from build123d import *

# Parameters (mm, degrees)
EXTRU_MINCE1_DEPTH      = 280
ESQUISSE2_R             = 1.5
ENL_V_MAT_EXTRU_1_DEPTH = 281.847489752
ESQUISSE3_R             = 1.5
ENL_V_MAT_EXTRU_2_DEPTH = 282.354758268
CONG_1_R                = 5


with BuildPart() as part:
    # Esquisse1 → Extru.-Mince1 (new body)
    with BuildSketch(Plane.XY):
        Polygon((-9.75, 19.5), (-9.75, 0), (9.75, 0), (9.75, 19.5), (8.25, 19.5), (8.25, 1.5), (-8.25, 1.5), (-8.25, 19.5), align=None)
    extrude(amount=EXTRU_MINCE1_DEPTH)

    # Esquisse2 → Enlèv. mat.-Extru.1 (cut, through all)
    with BuildSketch(Plane.XZ):
        with Locations(Location((0, 223, 0), (0, 0, 270))):
            Circle(ESQUISSE2_R)
        with Locations(Location((0, 205, 0), (0, 0, 270))):
            Circle(ESQUISSE2_R)
        with Locations(Location((0, 24, 0), (0, 0, 270))):
            Circle(ESQUISSE2_R)
        with Locations(Location((0, 174, 0), (0, 0, 270))):
            Circle(ESQUISSE2_R)
        with BuildLine():
            Line((-6, 280), (6, 280))
            Line((6, 280), (6, 264))
            ThreePointArc((6, 264), (4.828427125, 261.171572875), (2, 260))
            Line((2, 260), (-2, 260))
            ThreePointArc((-2, 260), (-4.828427125, 261.171572875), (-6, 264))
            Line((-6, 264), (-6, 280))
        make_face()
    extrude(amount=-ENL_V_MAT_EXTRU_1_DEPTH, mode=Mode.SUBTRACT)

    # Esquisse3 → Enlèv. mat.-Extru.2 (cut, through all)
    with BuildSketch(Plane(origin=(9.75, 0, 0), x_dir=(0, 0, -1), z_dir=(1, 0, 0))):
        with Locations(Location((-274, 7, 0), (0, 0, 90))):
            Circle(ESQUISSE3_R)
        with Locations(Location((-6, 13.5, 0), (0, 0, 90))):
            Circle(ESQUISSE3_R)
        Polygon((-280, 13.5), (-280, 19.5), (-245, 19.5), align=None)
    extrude(amount=-ENL_V_MAT_EXTRU_2_DEPTH, mode=Mode.SUBTRACT)

    # Congé1
    cong_1_edges = [part.edges().sort_by_distance(p)[0] for p in [
        (-9, 19.5, 0),
        (9, 19.5, 0),
    ]]
    fillet(cong_1_edges, radius=CONG_1_R)


solid = part.part
The model under review builds one solid part; all positions refer to its coordinate system, in mm. A direction names the side the tool comes from. Give positions to 0.01 mm unless a question says otherwise; leave off trailing zeros. Loops run counter-clockwise (first coordinate to the right, second up) from the corner with the lowest first, then second, coordinate; pieces in that order, holes last. Notation, with made-up numbers: (63.5, 51.25) -> (84.5, 51.25) arc R20 ccw to (84.5, 64.25) -> close; hole circle Ø3 at (76, 81). An arc over 180 degrees is marked (long way). Put each result on its own line as item: value. Start each with the question number.
1. We need section A-A on z = 132. State the section outline as (x, y) points, then the cut area to 4 significant figures.
2. Clearance check with flat-ended pins moving along their axes: P1, Ø4, axis at x = 0, z = 205, coming from the -Y side; P2, Ø4, axis at x = 0, z = 24, coming from the +Y side; P3, Ø0.8, axis at x = 0.5, y = 0.5, coming from the +Z side; P4, Ø2, axis at x = 7.5, y = 17.5, coming from the -Z side. State where each tip first meets the part, or that it passes through.
3. Wall thickness on probe 1 along X at (y, z) = (16, 48); probe 2 along Z at (x, y) = (9.1, 7); probe 3 along Y at (x, z) = (3.25, 112.5): over which ranges is each line inside the solid? List them lowest first.
4. For faces 5 (the face through (8.25, 11, 138)), 6 (the face through (0, 0, 138)), list the 3-axis set-ups (+Z, -Z, +X, -X, +Y, -Y) from which the entire face can be reached by the end or side of a thin tool; tool diameter is ignored.
5. Mouldability with a two-part tool opening along X and no side actions: class faces 1 (the face through (0, 1.5, 138)), 2 (the face through (-8.25, 10, 138)), 3 (the face through (-8.99, 16.54, 262.26)), 4 (the face through (9.75, 10, 138)) as released by +X, released by -X, zero draft, split by the parting line, or undercut.
Determined:
1. outline: (-9.75, 0) -> (9.75, 0) -> (9.75, 19.5) -> (8.25, 19.5) -> (8.25, 1.5) -> (-8.25, 1.5) -> (-8.25, 19.5) -> (-9.75, 19.5) -> close
1. area: 83.25 mm^2
2. P1: y = 0
2. P2: y = 1.5
2. P3: z = 260
2. P4: z = 0.58
3. probe 1: -9.75 to -8.25, 8.25 to 9.75
3. probe 2: 0 to 272.5, 275.5 to 280
3. probe 3: 0 to 1.5
4. face 5: +Z, -Z, +Y
4. face 6: +Z, -Z, +X, -X, -Y
5. face 1: undercut
5. face 2: undercut
5. face 3: zero draft
5. face 4: released by +X
